The model under review builds one solid part; all positions refer to its coordinate system, in mm. A direction names the side the tool comes from. Give positions to 0.01 mm unless a question says otherwise; leave off trailing zeros. Answer as CSV lines item,"result". Start each with the question number.
from build123d import *

# Parameters (mm, degrees)
F1_ANGLE  = 180
F2_R      = 31.5
F3_DEPTH  = 5
F4_W      = 15
F4_H      = 5
F5_DEPTH  = 10
F6_W      = 15
F6_H      = 5
F5_FACE_W = 15
F5_FACE_H = 5
F7_ANGLE  = 180


with BuildPart() as f1:
    # F0 (on Top) → F1 (revolve)
    with BuildSketch(Plane.XY):
        with BuildLine():
            ThreePointArc((0, -29.5), (20.85965, -20.85965), (29.5, 0))
            ThreePointArc((29.5, 0), (20.85965, 20.85965), (0, 29.5))
            Line((0, 29.5), (0, -29.5))
        make_face()
    revolve(axis=Axis((0, 0, 0), (0, -1, 0)), revolution_arc=F1_ANGLE)

    # F2 (on face) → F3 (join)
    with BuildSketch(Plane(origin=(0, 0, 0), x_dir=(1, 0, 0), z_dir=(0, 0, -1))):
        Circle(F2_R)
    extrude(amount=F3_DEPTH)

    # F4 (on face) → F5 (join)
    with BuildSketch(Plane(origin=(0, 0, -5), x_dir=(1, 0, 0), z_dir=(0, 0, -1))):
        with Locations((-17.5, 12.5)):
            Rectangle(F4_W, F4_H)
        with Locations((-17.5, -12.5)):
            Rectangle(F4_W, F4_H)
        with Locations((17.5, 12.5)):
            Rectangle(F4_W, F4_H)
        with Locations((17.5, -12.5)):
            Rectangle(F4_W, F4_H)
    extrude(amount=F5_DEPTH)

    # F6 (on face) + F5_face (on face) → F7 (revolve)
    with BuildSketch(Plane(origin=(0, 0, -15), x_dir=(1, 0, 0), z_dir=(0, 0, -1))):
        with Locations((-17.5, 12.5)):
            Rectangle(F6_W, F6_H)
    with BuildSketch(Plane(origin=(-17.5, -12.5, -15), x_dir=(1, 0, 0), z_dir=(0, 0, -1))):
        with Locations((35, 0)):
            Rectangle(F5_FACE_W, F5_FACE_H)
    revolve(axis=Axis((1.326716, 0, -15), (1, 0, 0)), revolution_arc=F7_ANGLE)


solid = f1.part
Item 1: Clearance check with flat-ended pins moving along their axes: pin 1 (7.5 mm diameter, centred on y = 7.5, z = -12, fed in from -X); pin 2 (5 mm diameter, centred on x = 18.5, z = -12.5, fed in from -Y); pin 3 (8 mm diameter, centred on x = -21, z = -12, fed in from +Y); pin 4 (2 mm diameter, centred on y = -2.5, z = -22.5, fed in from -X). State where each tip first meets the part, or that it passes through.
Item 2: For line 1 along X through (y, z) = (-10.5, -22); line 2 along Z through (x, y) = (19.5, -4.5); line 3 along Z through (x, y) = (-23.5, 3.5), list the stretches that pass through material, from the lowest coordinate up.
Item 3: Mouldability with a two-part tool opening along Y and no side actions: class faces 4 (the face through (17, 10, -10)), 5 (the face through (-4.101, -31.232, -2.465)), 6 (the face through (-10, -7, -23)) as released by +Y, released by -Y, zero draft, split by the parting line, or undercut.
Item 4: Machinability: for faces 1 (the face through (17, -10, -10)), 2 (the face through (-18, -15, -10)), 3 (the face through (-18, 15, -10)), which of the approach directions +Z, -Z, +X, -X, +Y, -Y give a long, thin tool a straight path to every point of the face, cutting with its end or side? Answer none if there is none.
Data:
1,pin 1,"stops at x = -25"
1,pin 2,"stops at y = -15"
1,pin 3,"stops at y = 15"
1,pin 4,"passes through"
2,line 1,"x = -25 to -10, 10 to 25"
2,line 2,"z = -29.31 to -23.93, -5 to 21.67"
2,line 3,"z = -29.59 to -24.37, -5 to 17.49"
3,face 4,"undercut"
3,face 5,"split by the parting line"
3,face 6,"zero draft"
4,face 1,"+X, -X"
4,face 2,"-Z, +X, -X, -Y"
4,face 3,"-Z, +X, -X, +Y"
